Check sheet for the modelled part. Datum: model origin and axes. Units: mm. A direction names the side the tool comes from. Give positions to 0.01 mm unless a question says otherwise; leave off trailing zeros. Order: outer loops, then holes, each group sorted by start corner. A loop starts at its lowest first (then second) coordinate and runs counter-clockwise, first axis right, second up. Notation, with made-up numbers: (64, 52.5) -> (112, 52.5) arc R16 ccw to (112, 80.5) -> close; hole circle Ø4 at (-8, 70). An arc over 180 degrees is marked (long way). Answer in a Markdown table with one row per item. Add a question column.
(1) Go/stop test with flat-tipped pins: pin 1 (4 mm diameter, centred on y = 5.15, z = 6, fed in from -X); pin 2 (1.2 mm diameter, centred on y = 3.5, z = 10.5, fed in from +X); pin 3 (4 mm diameter, centred on x = 26.5, z = 2.5, fed in from +Y). Record where each tip stops, or that it passes through.
(2) Set-up check for faces 1 (the face through (41.2, 5, 11)), 2 (the face through (41.2, 5, 1)), 3 (the face through (42.7, 2, 6)): record each of +Z, -Z, +X, -X, +Y, -Y from which the full face is reachable in a straight line by a thin tool's end or side.
(3) Cross-section at C-C (x = 33.5). Record the cut outline in (y, z).
(4) Cross-section at A-A (z = 6). Record the cut outline in (x, y).
(5) Release check for a two-part mould opening along Z. For faces 4 (the face through (21, 3, 0)), 5 (the face through (42, 5.5, 8.7)), 6 (the face through (21, 0, 6)), 7 (the face through (21.051, 3.842, 4.294)) record: released by +Z, released by -Z, zero draft, split by the parting line, or undercut.
(6) Cross-section at D-D (y = 0.75). Record the cut outline in (x, z), then the cut area to 3 significant figures.
(7) Thickness scan on L1, parallel to Y at x = 21, z = 6; L2, parallel to Z at x = 25.5, y = 5.15; L3, parallel to X at y = 3.25, z = 10.25. Record the ranges inside material, lowest first. Write a range as [from, to].
(8) Cross-section at B-B (y = 3.5). Record the cut outline in (x, z).
```python
from build123d import *

# Parameters (mm, degrees)
SKETCH1_W           = 41.2
SKETCH1_H           = 13
BOSS_EXTRUDE1_DEPTH = 12
BOSS_EXTRUDE3_DEPTH = 13
SKETCH2_R           = 2.15
CUT_EXTRUDE1_DEPTH  = 43.7
FILLET1_R           = 1


with BuildPart() as part:
    # Sketch1 → Boss-Extrude1 (new body)
    with BuildSketch(Plane.XY):
        with Locations((20.6, 6.5)):
            Rectangle(SKETCH1_W, SKETCH1_H)
    extrude(amount=BOSS_EXTRUDE1_DEPTH)

    # Sketch3 → Boss-Extrude3 (add)
    with BuildSketch(Plane(origin=(0, 13, 0), x_dir=(1, 0, 0), z_dir=(0, 1, 0))):
        Polygon((42.7, -8), (41.2, -9.5), (41.2, -2.5), (42.7, -4), align=None)
    extrude(amount=-BOSS_EXTRUDE3_DEPTH)

    # Sketch2 → Cut-Extrude1 (cut, through all)
    with BuildSketch(Plane.ZY):
        with Locations((6, 5.15)):
            Circle(SKETCH2_R)
        with BuildLine():
            Line((-1.89805103, 5.15), (0, 5.15))
            ThreePointArc((0, 5.15), (6, 11.15), (12, 5.15))
            Line((12, 5.15), (16.198164726, 5.15))
            Line((16.198164726, 5.15), (16.198164726, 14.318930959))
            Line((16.198164726, 14.318930959), (-1.89805103, 14.318930959))
            Line((-1.89805103, 14.318930959), (-1.89805103, 5.15))
        make_face()
    extrude(amount=-CUT_EXTRUDE1_DEPTH, mode=Mode.SUBTRACT)

    # Fillet1
    fillet1_edges = [part.edges().sort_by_distance(p)[0] for p in [
        (0, 2.575, 0),
        (0, 2.575, 12),
        (0, 11.15, 6),
    ]]
    fillet(fillet1_edges, radius=FILLET1_R)


solid = part.part
```
Answer below:
| question | item | result |
|---|---|---|
| 1 | pin 1 | passes through |
| 1 | pin 2 | stops at x = 41.2 |
| 1 | pin 3 | stops at y = 10.96 |
| 2 | face 1 | +Z, +X, +Y, -Y |
| 2 | face 2 | -Z, +X, +Y, -Y |
| 2 | face 3 | +Z, -Z, +X, +Y, -Y |
| 3 | outline | (0, 0) -> (5.15, 0) arc R6 ccw to (5.15, 12) -> (0, 12) -> close; hole circle Ø4.3 at (5.15, 6) |
| 4 | outline | (0, 0) -> (42.7, 0) -> (42.7, 3) -> (0, 3) -> close; (0, 7.3) -> (42.7, 7.3) -> (42.7, 11.15) -> (1, 11.15) arc R1 ccw to (0, 10.15) -> close |
| 5 | face 4 | released by -Z |
| 5 | face 5 | released by +Z |
| 5 | face 6 | zero draft |
| 5 | face 7 | undercut |
| 6 | outline | (0, 1) arc R1 ccw to (1, 0) -> (41.2, 0) -> (41.2, 2.5) -> (42.7, 4) -> (42.7, 8) -> (41.2, 9.5) -> (41.2, 12) -> (1, 12) arc R1 ccw to (0, 11) -> close |
| 6 | area | 502 mm² |
| 7 | L1 | y = [0, 3], [7.3, 11.15] |
| 7 | L2 | z = [0, 3.85], [8.15, 12] |
| 7 | L3 | x = [0, 41.2] |
| 8 | outline | (0, 1) arc R1 ccw to (1, 0) -> (41.2, 0) -> (41.2, 2.5) -> (42.7, 4) -> (42.7, 4.62) -> (0, 4.62) -> close; (0, 7.38) -> (42.7, 7.38) -> (42.7, 8) -> (41.2, 9.5) -> (41.2, 12) -> (1, 12) arc R1 ccw to (0, 11) -> close |
